Can you work these out from the model? Positions are in its coordinate system, mm. Coordinates: 2 decimals unless noted, no trailing zeros. Order: outer loops, then holes, each group sorted by start corner. A loop starts at its lowest first (then second) coordinate and runs counter-clockwise, first axis right, second up. Notation, with made-up numbers: M 49,80 L 66,80 A32 cw 66,109 Z; hole C 59,36 d2. An arc over 180 degrees is marked long. Answer as CSV lines item,"result". Start each with the question number.
1. Will these pins go through, and if not, where does the flat tip stop? pin 1 (10 mm diameter, centred on x = 22, y = 12, fed in from +Z); pin 2 (1.2 mm diameter, centred on y = 2, z = -2.5, fed in from -X); pin 3 (3 mm diameter, centred on x = -14, y = 14, fed in from +Z); pin 4 (2 mm diameter, centred on y = -23.5, z = -3, fed in from +X).
2. If we section it at A-A (y = 3): List the corners of the cut face in (x, z) for me.
3. I need wall thicknesses on line 1 along Y through (x, z) = (14, -3.55); line 2 along X through (y, z) = (-14, -3); line 3 along Y through (x, z) = (14, -1.15). Which ranges of each line are inside material? Lowest first, please. Write a range as from..to.
4. If we section it at B-B (y = -40): List the corners of the cut face in (x, z) for me.
```python
from build123d import *

# Parameters (mm, degrees)
EXTRUDE_START         = -4
SKETCH_1_R            = 1.65
SKETCH_1_R_2          = 1.1
EXTRUDE_266_DEPTH     = 4
CUT_EXTRUDE_START     = -4
SKETCH_2_W            = 32
SKETCH_2_H            = 66
CUT_EXTRUDE_347_DEPTH = 4
CUT_EXTRUDE_START_2   = -2
SKETCH_3_R            = 2
CUT_EXTRUDE_M2_DEPTH  = 2


with BuildPart() as part:
    # 草图1 → Extrude 266 (new body)
    with BuildSketch(Plane.XY.offset(EXTRUDE_START)):
        Polygon((-62, -50), (62, -50), (70, -42), (70, 42), (62, 50), (-62, 50), (-70, 42), (-70, -42), align=None)
        with Locations((-62, -40)):
            Circle(SKETCH_1_R, mode=Mode.SUBTRACT)
        with Locations((-14, -14)):
            Circle(SKETCH_1_R_2, mode=Mode.SUBTRACT)
        with Locations((-62, 40)):
            Circle(SKETCH_1_R, mode=Mode.SUBTRACT)
        with Locations((-14, 14)):
            Circle(SKETCH_1_R_2, mode=Mode.SUBTRACT)
        with Locations((62, -40)):
            Circle(SKETCH_1_R, mode=Mode.SUBTRACT)
        with Locations((14, -14)):
            Circle(SKETCH_1_R_2, mode=Mode.SUBTRACT)
        with Locations((62, 40)):
            Circle(SKETCH_1_R, mode=Mode.SUBTRACT)
        with Locations((14, 14)):
            Circle(SKETCH_1_R_2, mode=Mode.SUBTRACT)
        Polygon((-7, -10), (7, -10), (10, -7), (10, 7), (7, 10), (-7, 10), (-10, 7), (-10, -7), align=None, mode=Mode.SUBTRACT)
    extrude(amount=EXTRUDE_266_DEPTH)

    # 草图2 → Cut-Extrude 347 (cut)
    with BuildSketch(Plane.XY.offset(CUT_EXTRUDE_START)):
        with Locations((65, 0)):
            Rectangle(SKETCH_2_W, SKETCH_2_H)
        with Locations((-65, 0)):
            Rectangle(SKETCH_2_W, SKETCH_2_H)
    extrude(amount=CUT_EXTRUDE_347_DEPTH, mode=Mode.SUBTRACT)

    # 草图3 → M2头部内藏沉台 (cut)
    with BuildSketch(Plane.XY.offset(CUT_EXTRUDE_START_2)):
        with Locations((-14, -14)):
            Circle(SKETCH_3_R)
        with Locations((-14, 14)):
            Circle(SKETCH_3_R)
        with Locations((14, -14)):
            Circle(SKETCH_3_R)
        with Locations((14, 14)):
            Circle(SKETCH_3_R)
    extrude(amount=CUT_EXTRUDE_M2_DEPTH, mode=Mode.SUBTRACT)


solid = part.part
```
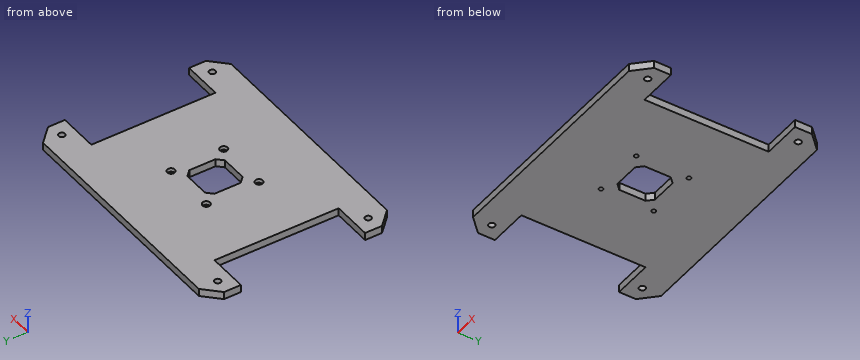
Solved:
1,pin 1,"z = 0"
1,pin 2,"x = -49"
1,pin 3,"z = -2"
1,pin 4,"x = 49"
2,outline,"M -49,-4 L -10,-4 L -10,0 L -49,0 Z; M 10,-4 L 49,-4 L 49,0 L 10,0 Z"
3,line 1,"-50..-15.1, -12.9..12.9, 15.1..50"
3,line 2,"-49..-15.1, -12.9..12.9, 15.1..49"
3,line 3,"-50..-16, -12..12, 16..50"
4,outline,"M -70,-4 L -63.65,-4 L -63.65,0 L -70,0 Z; M -60.35,-4 L 60.35,-4 L 60.35,0 L -60.35,0 Z; M 63.65,-4 L 70,-4 L 70,0 L 63.65,0 Z"
